```python
from build123d import *

# Parameters (mm, degrees)
F0_W         = 63.5
F0_H         = 25.4
F1_DEPTH     = 4.7625
F2_W         = 63.5
F2_H         = 16.51
F3_DEPTH     = 4.7625
F4_W         = 4.7625
F4_H         = 44.45
F5_DEPTH     = 63.5
F6_W         = 19.05
F6_H         = 4.7625
F7_DEPTH     = 63.5
F8_R         = 2.413
F9_DEPTH     = 4.7625
F10_R        = 5.08
F11_R        = 2.54
F12_T1_DEPTH = 76.2
F13_T1_DEPTH = 76.1003906189


# Not quite as in the source:
# - a fillet or chamfer that OpenCascade refuses, or shapes differently, is made with other operations: its cross-section is extruded or revolved along the edge and cut away or added


with BuildPart() as f1:
    # F0 (on Front) → F1 (new body)
    with BuildSketch(Plane.XZ):
        with Locations((-31.75, -12.7)):
            Rectangle(F0_W, F0_H)
    extrude(amount=F1_DEPTH)

    # F2 (on Top) → F3 (join)
    with BuildSketch(Plane.XY):
        with Locations((-31.75, -8.255)):
            Rectangle(F2_W, F2_H)
    extrude(amount=F3_DEPTH)

    # F4 (on Right) → F5 (join)
    with BuildSketch(Plane.YZ):
        with Locations((-14.12875, -22.225)):
            Rectangle(F4_W, F4_H)
    extrude(amount=-F5_DEPTH)

    # F6 (on Right) → F7 (join)
    with BuildSketch(Plane.YZ):
        with Locations((-26.035, -42.06875)):
            Rectangle(F6_W, F6_H)
    extrude(amount=-F7_DEPTH)

    # F8 (on face) → F9 (cut)
    with BuildSketch(Plane(origin=(0, 0, -44.45), x_dir=(1, 0, 0), z_dir=(0, 0, -1))):
        with Locations((-52.705, 26.035)):
            Circle(F8_R)
        with Locations((-38.735, 26.035)):
            Circle(F8_R)
        with Locations((-24.765, 26.035)):
            Circle(F8_R)
        with Locations((-10.795, 26.035)):
            Circle(F8_R)
    extrude(amount=-F9_DEPTH, mode=Mode.SUBTRACT)

    # F10
    f10_edges = [f1.edges().sort_by_distance(p)[0] for p in [
        (-31.75, 0, 4.7625),
        (-31.75, -16.51, 4.7625),
    ]]
    fillet(f10_edges, radius=F10_R)

    # F11
    f11_edges = [f1.edges().sort_by_distance(p)[0] for p in [
        (-31.75, -35.56, -39.6875),
    ]]
    fillet(f11_edges, radius=F11_R)

    # F12: fillet of radius 2.54 on 2 edges, made by hand

    # F12_s2 → F12_t1 (cut)
    with BuildSketch(Plane.YZ.offset(-69.85)):
        with BuildLine():
            ThreePointArc((-4.7625, -22.86), (-4.0185512242, -24.6560512242), (-2.2225, -25.4))
            Line((-2.2225, -25.4), (-4.7625, -25.4))
            Line((-4.7625, -25.4), (-4.7625, -22.86))
        make_face()
        with BuildLine():
            ThreePointArc((0, -22.86), (-0.7439487758, -24.6560512242), (-2.54, -25.4))
            Line((-2.54, -25.4), (0, -25.4))
            Line((0, -25.4), (0, -22.86))
        make_face()
    extrude(amount=F12_T1_DEPTH, mode=Mode.SUBTRACT)

    # F13: fillet of radius 2.54 on 1 edges, made by hand

    # F13_s2 → F13_t1 (cut)
    with BuildSketch(Plane.YZ.offset(-69.8001953095)):
        with BuildLine():
            ThreePointArc((-33.0399218762, -44.45), (-34.7199739587, -43.815), (-35.56, -42.2275))
            Line((-35.56, -42.2275), (-35.56, -44.45))
            Line((-35.56, -44.45), (-33.0399218762, -44.45))
        make_face()
    extrude(amount=F13_T1_DEPTH, mode=Mode.SUBTRACT)


solid = f1.part
```
Model file for the job. Use its own axes, mm. A direction names the side the tool comes from. Coordinates: 2 decimals unless noted, no trailing zeros. Order: outer loops, then holes, each group sorted by start corner. A loop starts at its lowest first (then second) coordinate and runs counter-clockwise, first axis right, second up. Notation, with made-up numbers: (62.5, -30) -> (98.5, -30) arc R25 ccw to (98.5, -11) -> close; hole circle Ø1 at (8.5, 29.5). An arc over 180 degrees is marked (long way). Answer as a JSON object with one key per item and string values. Group by question number.
1) Flat gauge pins, fed straight in: pin 1 (5.5 mm diameter, centred on x = -38.735, y = -26.035, fed in from +Z); pin 2 (13 mm diameter, centred on x = -39.5, y = -22.5, fed in from +Z); pin 3 (4 mm diameter, centred on x = -23.5, z = -8, fed in from -Y). Where does each tip first touch, or does it go through?
2) Cut at A-A, the plane z = -17.5. Write the cut outline in (x, y), then the cut area to 3 significant figures.
3) Pull direction Y, two halves, no side cores. Call faces 4 (the face through (-32.194, -34.796, -40.412)), 5 (the face through (-32.19, -4.09, -24.58)), 6 (the face through (-32, -8, 4.762)), 7 (the face through (-55.116, -26.141, -42.102)): +Y half, -Y half, draft (parallel to the pull), parting line (faces both ways), or undercut.
4) Cut at B-B, the plane x = -11.5. Write the cut outline in (y, z), then the cut area to 3 significant figures.
5) Cut at D-D, the plane x = -29. Write the cut outline in (y, z).
6) Drill centre lines: L1, parallel to Y at x = -35.5, z = -14; L2, parallel to Z at x = -48, y = -29.5; L3, parallel to Z at x = -5, y = -7. Where is each one in solid material? Low to high.
7) Which spindle directions (+Z, -Z, +X, -X, +Y, -Y) get a long thin tool onto all of the face, cutting with end or side? Do faces 1 (the face through (-32.19, -34.7, -43.83)), 2 (the face through (-31, -11.748, -23)), 3 (the face through (-31, -25, -39.688)). Say none if no direction does.
8) Cut at C-C, the plane y = -27.5. Write the cut outline in (x, z).
Check values:
{
 "1": {"pin 1": "stops at z = -39.69", "pin 2": "stops at z = 1.9", "pin 3": "stops at y = -16.51"},
 "2": {"outline": "(-63.5, -16.51) -> (0, -16.51) -> (0, -11.75) -> (-63.5, -11.75) -> close; (-63.5, -4.76) -> (0, -4.76) -> (0, 0) -> (-63.5, 0) -> close", "area": "605 mm²"},
 "3": {"face 4": "-Y half", "face 5": "undercut", "face 6": "draft", "face 7": "undercut"},
 "4": {"outline": "(-35.56, -42.23) arc R2.54 ccw to (-33.04, -44.45) -> (-28.34, -44.45) -> (-28.34, -39.69) -> (-33.02, -39.69) arc R2.54 ccw to start; (-23.73, -44.45) -> (-11.75, -44.45) -> (-11.75, 0) -> (-4.76, 0) -> (-4.76, -22.86) arc R2.54 ccw to (-2.38, -25.4) arc R2.54 ccw to (0, -22.86) -> (0, -0.32) arc R5.08 ccw to (-5.08, 4.76) -> (-11.43, 4.76) arc R5.08 ccw to (-16.51, -0.32) -> (-16.51, -39.69) -> (-23.73, -39.69) -> close", "area": "463 mm²"},
 "5": {"outline": "(-35.56, -42.23) arc R2.54 ccw to (-33.04, -44.45) -> (-11.75, -44.45) -> (-11.75, 0) -> (-4.76, 0) -> (-4.76, -22.86) arc R2.54 ccw to (-2.38, -25.4) arc R2.54 ccw to (0, -22.86) -> (0, -0.32) arc R5.08 ccw to (-5.08, 4.76) -> (-11.43, 4.76) arc R5.08 ccw to (-16.51, -0.32) -> (-16.51, -39.69) -> (-33.02, -39.69) arc R2.54 ccw to start"},
 "6": {"L1": "y = -16.51 to -11.75, -4.76 to 0", "L2": "z = -44.45 to -39.69", "L3": "z = 0 to 4.76"},
 "7": {"face 1": "-Z, +X, -X, -Y", "face 2": "-Z, +X, -X", "face 3": "+Z, +X, -X, -Y"},
 "8": {"outline": "(-63.5, -44.45) -> (-54.62, -44.45) -> (-54.62, -39.69) -> (-63.5, -39.69) -> close; (-50.79, -44.45) -> (-40.65, -44.45) -> (-40.65, -39.69) -> (-50.79, -39.69) -> close; (-36.82, -44.45) -> (-26.68, -44.45) -> (-26.68, -39.69) -> (-36.82, -39.69) -> close; (-22.85, -44.45) -> (-12.71, -44.45) -> (-12.71, -39.69) -> (-22.85, -39.69) -> close; (-8.88, -44.45) -> (0, -44.45) -> (0, -39.69) -> (-8.88, -39.69) -> close"}
}
